Geometry: final body of the model. Coordinates: model frame, mm. A direction names the side the tool comes from. Give positions to 0.01 mm unless a question says otherwise; leave off trailing zeros. Write each loop counter-clockwise with the first axis right and the second up, starting at its lowest first coordinate (ties: lowest second). Pieces come first, ordered by that corner, then holes. Notation, with made-up numbers: M 11,33 L 33,33 A22 cw 33,49 Z; hole C 51,22.5 d9. An arc over 180 degrees is marked long. Answer as a JSON object with one key per item and string values.
from build123d import *

# Parameters (mm, degrees)
SKETCH1_R           = 1.5
BOSS_EXTRUDE1_DEPTH = 50
SKETCH2_R           = 4
BOSS_EXTRUDE2_DEPTH = 3
BOSS_EXTRUDE3_DEPTH = 3
SKETCH5_W           = 4.5
SKETCH5_H           = 3
CUT_EXTRUDE1_DEPTH  = 4
FILLET1_R           = 2


with BuildPart() as part:
    # Sketch1 → Boss-Extrude1 (new body)
    with BuildSketch(Plane(origin=(0, 0, 0), x_dir=(1, 0, 0), z_dir=(0, 1, 0))):
        Circle(SKETCH1_R)
    extrude(amount=BOSS_EXTRUDE1_DEPTH)

    # Sketch2 → Boss-Extrude2 (add)
    with BuildSketch(Plane(origin=(0, 0, 0), x_dir=(-1, 0, 0), z_dir=(0, -1, 0))):
        Circle(SKETCH2_R)
    extrude(amount=BOSS_EXTRUDE2_DEPTH)

    # Sketch4 → Boss-Extrude3 (add)
    with BuildSketch(Plane.XY.offset(1.5)):
        Polygon((0, 50), (6, 50), (6, 59), (-6, 59), (-6, 50), align=None)
    extrude(amount=-BOSS_EXTRUDE3_DEPTH)

    # Sketch5 → Cut-Extrude1 (cut)
    with BuildSketch(Plane.XY.offset(1.5)):
        with Locations((-2.25, 54.5)):
            Rectangle(SKETCH5_W, SKETCH5_H)
        with Locations((2.25, 54.5)):
            Rectangle(SKETCH5_W, SKETCH5_H)
    extrude(amount=-CUT_EXTRUDE1_DEPTH, mode=Mode.SUBTRACT)

    # Fillet1
    fillet1_edges = [part.edges().sort_by_distance(p)[0] for p in [
        (6, 50, 0),
        (-6, 50, 0),
        (-6, 59, 0),
        (6, 59, 0),
    ]]
    fillet(fillet1_edges, radius=FILLET1_R)


solid = part.part
1) Contact query for flat-ended pins moving along their axis: P1, Ø7, axis at x = -1, y = 54, coming from the +Z side; P2, Ø2.5, axis at x = 2.5, y = 56, coming from the -Z side. Output: stop coordinate, or through.
Geometry check:
{"P1": "stops at z = 1.5", "P2": "stops at z = -1.5"}
2) Cut plane C-C on x = 2.5. Return loops of the section in (y, z).
Geometry check:
{"outline": "M -3,-3.12 L 0,-3.12 L 0,3.12 L -3,3.12 Z; M 50,-1.5 L 53,-1.5 L 53,1.5 L 50,1.5 Z; M 56,-1.5 L 59,-1.5 L 59,1.5 L 56,1.5 Z"}
3) Pull-direction query (X, two-part tool) for faces 1 (the flat face through (4.5, 54, 0)), 2 (the flat face through (-6, 55, 0)), 3 (the flat face through (-2, 0, 0)); classes: pulls with the +X half, pulls with the -X half, needs draft (parallel to the pull), parting line crosses it, or undercut.
Geometry check:
{"face 1": "undercut", "face 2": "pulls with the -X half", "face 3": "needs draft"}
4) Line query: line 1 (Y direction, x = 0.25, z = 0.5); line 2 (Y direction, x = -4, z = 0.5); line 3 (Y direction, x = -1, z = -2.5). Output: solid intervals per line, ascending. Write a range as from..to.
Geometry check:
{"line 1": "y = -3..53, 56..59", "line 2": "y = 50..53, 56..59", "line 3": "y = -3..0"}
5) Set-up query: faces 4 (the cylindrical face through (-1.5, 24.65, -0.07)), 5 (the flat face through (0, -3, 0)), 6 (the flat face through (-0.1, 52.6, 1.5)), 7 (the cylindrical face through (0.867, -1.479, 3.905)), 8 (the flat face through (0, 53, 0)). Return all of +Z, -Z, +X, -X, +Y, -Y with unobstructed straight access to the full face (end or side cutting, diameter ignored); none if empty.
Geometry check:
{"face 4": "none", "face 5": "+Z, -Z, +X, -X, -Y", "face 6": "+Z, +X, -X, +Y", "face 7": "-Y", "face 8": "+Z, -Z"}
6) Cut plane B-B on z = 0. Return loops of the section in (x, y).
Geometry check:
{"outline": "M -6,52 A2 ccw -4,50 L -1.5,50 L -1.5,0 L -4,0 L -4,-3 L 4,-3 L 4,0 L 1.5,0 L 1.5,50 L 4,50 A2 ccw 6,52 L 6,57 A2 ccw 4,59 L -4,59 A2 ccw -6,57 Z; hole M -4.5,53 L 4.5,53 L 4.5,56 L -4.5,56 Z"}
7) Cut plane A-A on y = 54.5. Return loops of the section in (x, z), and give its area (3 significant figures).
Geometry check:
{"outline": "M -6,-1.5 L -4.5,-1.5 L -4.5,1.5 L -6,1.5 Z; M 4.5,-1.5 L 6,-1.5 L 6,1.5 L 4.5,1.5 Z", "area": "9.00 mm2"}
8) Cut plane D-D on y = 9.5. Return loops of the section in (x, z).
Geometry check:
{"outline": "C 0,0 d3"}
